Autodesk Inventor part; units mm, degrees
ref_plane "YZ Plane" through (0, 0, 0) normal (1, 0, 0) x (0, 1, 0)
ref_plane "XZ Plane" through (0, 0, 0) normal (0, 1, 0) x (-1, 0, 0)
ref_plane "XY Plane" through (0, 0, 0) normal (0, 0, 1) x (1, 0, 0)
sketch "Esquisse1" plane through (0, 0, 0) normal (0, 1, 0) x (-1, 0, 0)
  line L0 (56.6857, 276.3714) -> (-55.3143, 276.3714)
  line L1 (-55.3143, 276.3714) -> (-55.3143, -142.6286)
  line L2 (-55.3143, -142.6286) -> (56.6857, -142.6286)
  line L3 (56.6857, -142.6286) -> (56.6857, 276.3714)
  point P0 (0, 0)
  dimension "d0" = 112
  dimension "d1" = 419
extrude "Extrusion1" add sketch "Esquisse1" along normal blind 22
sketch "Esquisse2" plane through (0, 22, 0) normal (0, 1, 0) x (1, 0, 0)
  line L0 (-56.6857, 142.6286) -> (-56.6857, -276.3714)
  line L1 (55.3143, -276.3714) -> (55.3143, 142.6286)
  line L2 (-56.6857, -276.3714) -> (55.3143, -276.3714)
  line L3 (55.3143, -276.3714) -> (55.3143, -254.3714)
  line L4 (55.3143, -254.3714) -> (-56.6857, -254.3714)
  line L5 (-56.6857, -254.3714) -> (-56.6857, -276.3714)
  line L6 (55.3143, 142.6286) -> (-56.6857, 142.6286)
  line L7 (-56.6857, 142.6286) -> (55.3143, 142.6286)
  line L8 (55.3143, 142.6286) -> (55.3143, 120.6286)
  line L9 (55.3143, 120.6286) -> (-56.6857, 120.6286)
  line L10 (-56.6857, 120.6286) -> (-56.6857, 142.6286)
  line L11 (-56.6857, -254.3714) -> (-34.6857, -254.3714)
  line L12 (-34.6857, -254.3714) -> (-34.6857, 120.6286)
  line L13 (-34.6857, 120.6286) -> (-56.6857, 120.6286)
  line L14 (-56.6857, 120.6286) -> (-56.6857, -254.3714)
  point P0 (0, 0)
  dimension "d4" = 22
  dimension "d5" = 22
  dimension "d6" = 22
extrude "Extrusion2" add sketch "Esquisse2" along normal blind 55 contours L6 L1 L9 L0 | L9 L12 L4 L0 | L4 L1 L2 L0
sketch "Esquisse3" plane through (0, 22, 0) normal (0, 1, 0) x (1, 0, 0)
  line L0 (-34.6857, 120.6286) -> (-34.6857, -254.3714)
  line L1 (-34.6857, 120.6286) -> (55.3143, 120.6286)
  line L2 (-34.6857, -254.3714) -> (55.3143, -254.3714)
  line L3 (55.3143, -254.3714) -> (55.3143, 120.6286)
  line L4 (55.3143, 120.6286) -> (-34.6857, 120.6286)
  line L5 (-34.6857, 120.6286) -> (-34.6857, -254.3714)
  circle A0 centre (10.3143, 83.1286) radius 28
  circle A1 centre (10.3143, 8.1286) radius 28
  circle A2 centre (10.3143, -66.8714) radius 28
  circle A3 centre (10.3143, -141.8714) radius 28
  circle A4 centre (10.3143, -216.8714) radius 28
  point P0 (0, 0)
  dimension "d9" = 37.5
  dimension "d10" = 45
  dimension "d11" = 56
  dimension "d12" = 75
  dimension "d13" = 56
  dimension "d14" = 45
  dimension "d15" = 56
  dimension "d16" = 45
  dimension "d17" = 75
  dimension "d18" = 56
  dimension "d19" = 45
  dimension "d20" = 75
  dimension "d21" = 45
  dimension "d22" = 75
  dimension "d23" = 56
extrude "Extrusion3" add sketch "Esquisse3" along normal blind 3
properties part number "conteneur-boues"
Verification items for the finished model (mm, model axes). A direction names the side the tool comes from. Coordinates: 2 decimals unless noted, no trailing zeros. Write each loop counter-clockwise with the first axis right and the second up, starting at its lowest first coordinate (ties: lowest second). Pieces come first, ordered by that corner, then holes. Notation, with made-up numbers: M -36.5,86 L 2.5,86 A15 ccw 2.5,101 Z; hole C 54,30 d2. An arc over 180 degrees is marked long. One line per question, with ' | ' between items.
1) Material ranges on L1, parallel to Z at x = 50, y = 48; L2, parallel to X at y = 61.5, z = 71; L3, parallel to Y at x = -29, z = -73, recorded low to high.
Solutions:
L1: -142.63 to -120.63, 254.37 to 276.37 | L2: -56.69 to -34.69 | L3: 0 to 25
2) Access from +Z, -Z, +X, -X, +Y, -Y to the whole of each face (thin tool, end or side, straight path). Record for faces 1 (the face through (-38, 77, 19)), 2 (the face through (11, 22, 217)), 3 (the face through (-20, 25, 64)).
Solutions:
face 1: +Z, -Z, +X, -X, +Y | face 2: +Y | face 3: +X, +Y
3) Sectioned sample at B-B on x = -26.5. Record the cut outline in (y, z), then the cut area to 3 significant figures.
Solutions:
outline: M 0,-142.63 L 77,-142.63 L 77,-120.63 L 25,-120.63 L 25,254.37 L 77,254.37 L 77,276.37 L 0,276.37 Z | area: 12,800 mm^2
4) Depth check by flat-ended pin: pin 1 Ø3 at (x, z) = (-23.5, 213.5) entering from +Y; pin 2 Ø17 at (x, z) = (-1, -4.5) entering from +Y; pin 3 Ø3 at (y, z) = (53.5, 224.5) entering from +X. Enter the tip coordinate at first touch or a pass-through.
Solutions:
pin 1: y = 25 | pin 2: y = 22 | pin 3: x = -34.69
5) Sectioned sample at C-C on z = 104. Record the cut outline in (x, y).
Solutions:
outline: M -56.69,0 L 55.31,0 L 55.31,25 L -34.69,25 L -34.69,77 L -56.69,77 Z
6) Sectioned sample at A-A on y = 69.5. Record the cut outline in (x, z), then the cut area to 3 significant figures.
Solutions:
outline: M -56.69,-142.63 L 55.31,-142.63 L 55.31,-120.63 L -34.69,-120.63 L -34.69,254.37 L 55.31,254.37 L 55.31,276.37 L -56.69,276.37 Z | area: 13,200 mm^2
7) Sectioned sample at D-D on x = -7. Record the cut outline in (y, z), then the cut area to 3 significant figures.
Solutions:
outline: M 0,-142.63 L 77,-142.63 L 77,-120.63 L 25,-120.63 L 25,-105.13 L 22,-105.13 L 22,-61.12 L 25,-61.12 L 25,-30.13 L 22,-30.13 L 22,13.88 L 25,13.88 L 25,44.87 L 22,44.87 L 22,88.88 L 25,88.88 L 25,119.87 L 22,119.87 L 22,163.88 L 25,163.88 L 25,194.87 L 22,194.87 L 22,238.88 L 25,238.88 L 25,254.37 L 77,254.37 L 77,276.37 L 0,276.37 Z | area: 12,100 mm^2
